Here's how the part is built. I have some questions about the finished solid (model axes, mm). Face numbers are marked on the shaded views. A direction names the side the tool comes from. Coordinates: 2 decimals unless noted, no trailing zeros. Write each loop counter-clockwise with the first axis right and the second up, starting at its lowest first coordinate (ties: lowest second). Pieces come first, ordered by that corner, then holes.
Item 1: If we mould it in two halves opening along Y, with no side actions, what happens to the marked faces 4, 5 and 6? For each: pulls with the +Y half, pulls with the -Y half, needs draft (parallel to the pull), parting line crosses it, or undercut.
Item 2: I want a section at A-A (x = 15). Please give me the cut outline in (y, z), and give its area (3 significant figures).
Item 3: Please list where these lines run through material, in increasing order: line 1 (X direction, y = 0, z = -0.75); line 2 (X direction, y = 3, z = 0); line 3 (X direction, y = -13, z = 0.5).
Item 4: I want a section at B-B (z = -3.5). Please give me the cut outline in (x, y).
Item 5: For the marked faces 1, 2 and 3, which set-ups out of +Z, -Z, +X, -X, +Y, -Y let a thin tool reach every point of the face, with its end or its side?
Item 6: I want a section at D-D (x = 0). Please give me the cut outline in (y, z).
Item 7: I want a section at C-C (y = -9.5). Please give me the cut outline in (x, z) (3 decimals), and give its area (3 significant figures).
Item 8: I'm going to push flat-ended pins straight in: P1, Ø5, axis at y = -3, z = 2, coming from the +X side; P2, Ø5.5, axis at x = 9.5, y = 0, coming from the +Z side; P3, Ø2, axis at y = -14, z = -3, coming from the -X side. Where does each tip first touch, or does it pass through?
from build123d import *

# Parameters (mm, degrees)
BOSS_EXTRUDE1_DEPTH                             = 5
CSK_FOR_M3_FLAT_HEAD_MACHINE_SCREW1_D           = 3.4
CSK_FOR_M3_FLAT_HEAD_MACHINE_SCREW1_DEPTH       = 15.4
CSK_FOR_M3_FLAT_HEAD_MACHINE_SCREW1_CSINK_D     = 6.3
CSK_FOR_M3_FLAT_HEAD_MACHINE_SCREW1_CSINK_ANGLE = 90
CSK_FOR_M3_FLAT_HEAD_MACHINE_SCREW1_TIP         = 1.041353257
F_3_0MM_DOWEL_HOLE1_D                           = 3


with BuildPart() as part:
    # Sketch2 → Boss-Extrude1 (new, symmetric)
    with BuildSketch(Plane.XY):
        Polygon((-14.5, -15.2), (-14.5, 15.2), (-17.5, 15.2), (-17.5, 20.2), (17.5, 20.2), (17.5, 15.2), (14.5, 15.2), (14.5, -15.2), (17.5, -15.2), (17.5, -20.2), (-17.5, -20.2), (-17.5, -15.2), align=None)
    extrude(amount=BOSS_EXTRUDE1_DEPTH, both=True)

    # CSK for M3 Flat Head Machine Screw1
    with Locations(Plane(origin=(-9.5, 0, 5), x_dir=(1, 0, 0), z_dir=(0, 0, 1))):
        with Locations((0, 0), (9.5, 9.5), (19, 0), (9.5, -9.5)):
            CounterSinkHole(CSK_FOR_M3_FLAT_HEAD_MACHINE_SCREW1_D / 2, CSK_FOR_M3_FLAT_HEAD_MACHINE_SCREW1_CSINK_D / 2, depth=CSK_FOR_M3_FLAT_HEAD_MACHINE_SCREW1_DEPTH, counter_sink_angle=CSK_FOR_M3_FLAT_HEAD_MACHINE_SCREW1_CSINK_ANGLE)
            with Locations((0, 0, -(CSK_FOR_M3_FLAT_HEAD_MACHINE_SCREW1_DEPTH + CSK_FOR_M3_FLAT_HEAD_MACHINE_SCREW1_TIP / 2))):  # 117.02° drill point
                Cone(0, CSK_FOR_M3_FLAT_HEAD_MACHINE_SCREW1_D / 2, CSK_FOR_M3_FLAT_HEAD_MACHINE_SCREW1_TIP, mode=Mode.SUBTRACT)

    # Ø3.0mm Dowel Hole1 (through all)
    with Locations(Plane(origin=(0, 20.2, 0), x_dir=(1, 0, 0), z_dir=(0, 1, 0))):
        with Locations((-4.75, 0.725), (4.75, 0.725)):
            Hole(F_3_0MM_DOWEL_HOLE1_D / 2)


solid = part.part
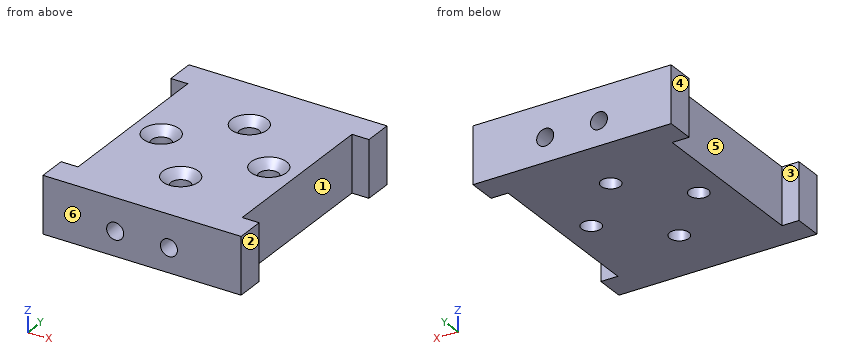
Answer:
1. face 4: needs draft
1. face 5: undercut
1. face 6: pulls with the -Y half
2. outline: (-20.2, -5) - (-15.2, -5) - (-15.2, 5) - (-20.2, 5) - close; (15.2, -5) - (20.2, -5) - (20.2, 5) - (15.2, 5) - close
2. area: 100 mm2
3. line 1: x = -14.5 to -11.2, -7.8 to -6.25, -3.25 to 3.25, 6.25 to 7.8, 11.2 to 14.5
3. line 2: x = -14.5 to -6.06, -3.44 to 3.44, 6.06 to 14.5
3. line 3: x = -14.5 to -5.62, -3.88 to 3.88, 5.62 to 14.5
4. outline: (-17.5, -20.2) - (17.5, -20.2) - (17.5, -15.2) - (14.5, -15.2) - (14.5, 15.2) - (17.5, 15.2) - (17.5, 20.2) - (-17.5, 20.2) - (-17.5, 15.2) - (-14.5, 15.2) - (-14.5, -15.2) - (-17.5, -15.2) - close; hole circle Ø3.4 at (-9.5, 0); hole circle Ø3.4 at (0, -9.5); hole circle Ø3.4 at (0, 9.5); hole circle Ø3.4 at (9.5, 0)
5. face 1: +Z, -Z, +X
5. face 2: +Z, -Z, +X, +Y, -Y
5. face 3: +Z, -Z, -X
6. outline: (-20.2, -5) - (-11.2, -5) - (-11.2, 3.55) - (-12.65, 5) - (-20.2, 5) - close; (-7.8, -5) - (7.8, -5) - (7.8, 3.55) - (6.35, 5) - (-6.35, 5) - (-7.8, 3.55) - close; (11.2, -5) - (20.2, -5) - (20.2, 5) - (12.65, 5) - (11.2, 3.55) - close
7. outline: (-14.5, -5) - (-1.7, -5) - (-1.7, 3.55) - (-3.15, 5) - (-14.5, 5) - close; (1.7, -5) - (14.5, -5) - (14.5, 5) - (3.15, 5) - (1.7, 3.55) - close; hole circle Ø3 at (-4.75, -0.725); hole circle Ø3 at (4.75, -0.725)
7. area: 240 mm2
8. P1: stops at x = 14.5
8. P2: stops at z = 4.6
8. P3: stops at x = -14.5
